```python
from build123d import *

# Parameters (mm, degrees)
SKETCH2_R           = 5
BOSS_EXTRUDE2_DEPTH = 57
SKETCH2_5_R         = 54
BOSS_EXTRUDE4_DEPTH = 11
SKETCH3_R           = 4
BOSS_EXTRUDE6_DEPTH = 10


with BuildPart() as part:
    # Sketch2 → Boss-Extrude2 (new body)
    with BuildSketch(Plane(origin=(0, 0, 0), x_dir=(1, 0, 0), z_dir=(0, 1, 0))):
        with Locations(Location((0, 0, 0), (0, 0, 270))):
            Circle(SKETCH2_R)
    extrude(amount=-BOSS_EXTRUDE2_DEPTH)

    # Sketch2_5 → Boss-Extrude4 (add)
    with BuildSketch(Plane(origin=(0, 0, 0), x_dir=(1, 0, 0), z_dir=(0, 1, 0))):
        with Locations(Location((0, 0, 0), (0, 0, 270))):
            Circle(SKETCH2_5_R)
    extrude(amount=BOSS_EXTRUDE4_DEPTH)

    # Sketch3 → Boss-Extrude6 (add)
    with BuildSketch(Plane.XZ):
        with Locations(Location((-46, 19, 0), (0, 0, 90))):
            Circle(SKETCH3_R)
        with BuildLine():
            ThreePointArc((-28.565713714, -28), (36.878177829, -15.491933385), (0, 40))
            add(Edge.make_bspline(
                [(-28.565713714, -28), (-4.359091078, 1.635688794), (0, 40)],
                knots=[0, 0, 0, 1, 1, 1], degree=2))
        make_face()
    extrude(amount=BOSS_EXTRUDE6_DEPTH)


solid = part.part
```
Model file for the job. Use its own axes, mm. A direction names the side the tool comes from. Coordinates: 2 decimals unless noted, no trailing zeros. Write each loop counter-clockwise with the first axis right and the second up, starting at its lowest first coordinate (ties: lowest second). Pieces come first, ordered by that corner, then holes. Notation, with made-up numbers: (53.5, 30.5) - (66.5, 30.5) arc R13 cw to (66.5, 48.5) - close; hole circle Ø5 at (53.5, 30.5). An arc over 180 degrees is marked (long way). One line per question, with ' | ' between items. Start each with the question number.
Q1. Pull direction Z, two halves, no side cores. Call faces 1 (the face through (-46, -10, 19)), 2 (the face through (-52.716, 5.423, -11.706)): pulls with the +Z half, pulls with the -Z half, needs draft (parallel to the pull), parting line crosses it, or undercut.
Q2. Cut at D-D, the plane x = -46. List the corners of the cut face in (y, z).
Q3. Cut at A-A, the plane x = 24. List the corners of the cut face in (y, z), then the cut area to 3 significant figures.
Q4. Drill centre lines: line 1 (Y direction, x = 1, z = 22); line 2 (Y direction, x = 47, z = -22.5); line 3 (X direction, y = 8, z = -27). Where is each one in solid material? Low to high. Write a range as [from, to].
Q5. Cut at B-B, the plane y = 2. List the corners of the cut face in (x, z).
Q6. 3-axis set-ups, long thin cutter, end or side, ignore diameter. For faces 3 (the face through (0, -57, 0)), 4 (the face through (-43.6, -4.9, 15.8)): which of +Z, -Z, +X, -X, +Y, -Y reach the whole face in a straight line?
Q7. Pin check, flat tips, straight feed: pin 1 (6 mm diameter, centred on x = -16, z = 42, fed in from -Y); pin 2 (20.5 mm diameter, centred on x = 22.5, z = 8.5, fed in from -Y); pin 3 (12 mm diameter, centred on x = -12.5, y = -50, fed in from +Z); pin 4 (10 mm diameter, centred on y = -2.5, z = -23.5, fed in from +X). Stop position of each tip, or through.
Q8. Cut at C-C, the plane y = -12. List the corners of the cut face in (x, z).
Answer below:
1) face 1: needs draft | face 2: parting line crosses it
2) outline: (-10, 15) - (0, 15) - (0, -28.28) - (11, -28.28) - (11, 28.28) - (0, 28.28) - (0, 23) - (-10, 23) - close
3) outline: (-10, -32) - (0, -32) - (0, -48.37) - (11, -48.37) - (11, 48.37) - (0, 48.37) - (0, 32) - (-10, 32) - close | area: 1,700 mm^2
4) line 1: [-10, 11] | line 2: [0, 11] | line 3: [-46.77, 46.77]
5) outline: circle Ø108 at (0, 0)
6) face 3: +Z, -Z, +X, -X, -Y | face 4: -Y
7) pin 1: y = 0 | pin 2: y = -10 | pin 3: through | pin 4: x = 50.48
8) outline: circle Ø10 at (0, 0)
